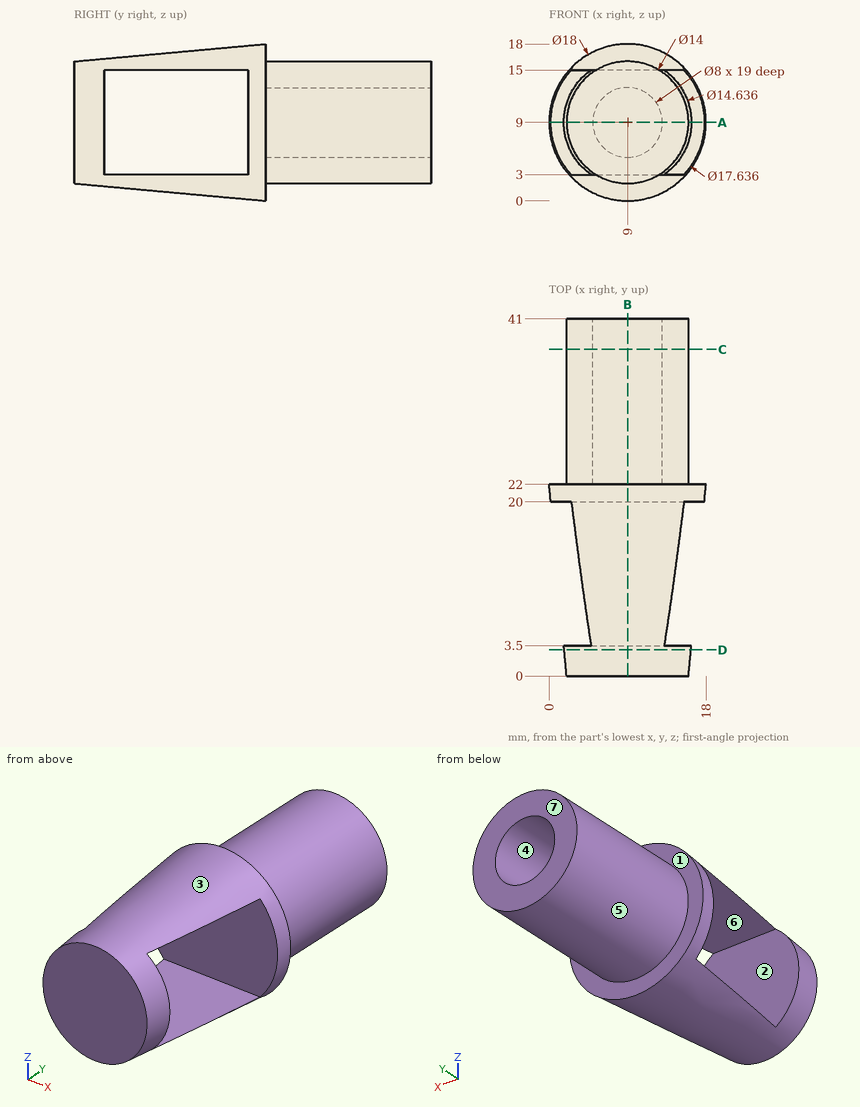
For this review, use the dimensioned drawing (mm, ordinates from the lowest corner) and the shaded views. A direction names the side the tool comes from. Coordinates: 2 decimals unless noted, no trailing zeros. Loops run counter-clockwise (first coordinate to the right, second up) from the corner with the lowest first, then second, coordinate; pieces in that order, holes last. Notation, with made-up numbers: (13.25, 35) - (52.25, 35) arc R17 ccw to (52.25, 47) - close; hole circle Ø11 at (31, -14.5). An arc over 180 degrees is marked (long way). Use CSV: the item, a comma, the result in double quotes. Start each with the question number.
1) The part is to be moulded in two halves that separate along Z. For the marked faces 4, 5, 6 and 7, say which applies: +Z half, -Z half, draft (parallel to the pull), parting line (faces both ways), or undercut.
2) For pin 1 Ø10.5 at (x, y) = (10.5, 11.5) entering from +Z; pin 2 Ø1 at (y, z) = (30.5, 6.5) entering from +X; pin 3 Ø8 at (y, z) = (30.5, 11.5) entering from -X, all flat-tipped, find the tip position at first contact; note any pin that passes through.
3) Consider section C-C on y = 37.5. Write out the cut boundary in (x, z).
4) Consider section A-A on z = 9. Write out the cut boundary in (x, y).
5) Wall thickness on L1, parallel to X at y = 36.5, z = 9; L2, parallel to Y at x = 8.5, z = 11; L3, parallel to Y at x = 10.75, z = 14: over which ranges is each line inside the solid? List them lowest first. Write a range as from..to.
6) Tool access review of the marked faces 1, 2 and 3: name each direction out of +Z, -Z, +X, -X, +Y, -Y from which nothing blocks a thin tool from reaching the whole face with its end or side.
7) Consider section D-D on y = 3. Write out the cut boundary in (x, z) (1 decimal).
8) Consider section B-B on x = 9. Write out the cut boundary in (y, z), then the cut area to 3 significant figures.
Geometry says:
1,face 4,"undercut"
1,face 5,"parting line"
1,face 6,"undercut"
1,face 7,"draft"
2,pin 1,"z = 17.51"
2,pin 2,"x = 15.71"
2,pin 3,"x = 2"
3,outline,"circle Ø14 at (9, 9); hole circle Ø8 at (9, 9)"
4,outline,"(0, 22) - (0.18, 20) - (17.82, 20) - (18, 22) - (16, 22) - (16, 41) - (13, 41) - (13, 22) - (5, 22) - (5, 41) - (2, 41) - (2, 22) - close; (1.68, 3.5) - (2, 0) - (16, 0) - (16.32, 3.5) - close"
5,L1,"2..5, 13..16"
5,L2,"0..3.5, 20..22"
5,L3,"0..3.5, 20..41"
6,face 1,"+Y"
6,face 2,"+X, -X"
6,face 3,"-Y"
7,outline,"circle Ø14.5 at (9, 9)"
8,outline,"(0, 2) - (22, 0) - (22, 2) - (41, 2) - (41, 5) - (22, 5) - (22, 13) - (41, 13) - (41, 16) - (22, 16) - (22, 18) - (0, 16) - close; hole (3.5, 3) - (20, 3) - (20, 15) - (3.5, 15) - close"
8,area,"268 mm^2"
